Autodesk Inventor part; units mm, degrees
ref_plane "YZ Plane" through (0, 0, 0) normal (1, 0, 0) x (0, 1, 0)
ref_plane "XZ Plane" through (0, 0, 0) normal (0, 1, 0) x (-1, 0, 0)
ref_plane "XY Plane" through (0, 0, 0) normal (0, 0, 1) x (1, 0, 0)
sketch "Sketch1" plane through (0, 0, 0) normal (0, 1, 0) x (-1, 0, 0)
  circle A0 centre (59.0549, -74.4145) radius 1.6
  circle A1 centre (-59.0549, -74.4145) radius 1.6
  line L0 (57.79, -78.2092) -> (0, -58.9459)
  line L1 (-57.79, -78.2092) -> (0, -58.9459)
  line L2 (-60.3198, -70.6198) -> (0, -50.5132)
  line L3 (60.3198, -70.6198) -> (0, -50.5132)
  arc A2 (57.79, -78.2092) -> (60.3198, -70.6198) centre (59.0549, -74.4145) ccw
  arc A3 (-60.3198, -70.6198) -> (-57.79, -78.2092) centre (-59.0549, -74.4145) ccw
extrude "Extrusion1" add sketch "Sketch1" along normal blind 45
properties part number "Front Support"
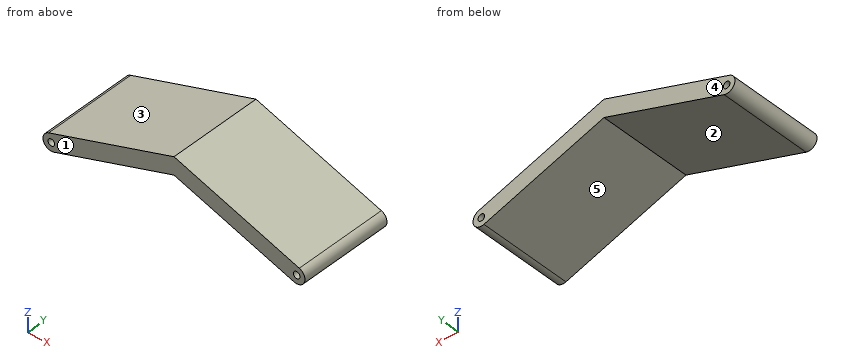
Design review of the part built by this model. Coordinates are the model's own, in mm. Face numbers are marked on the shaded views. A direction names the side the tool comes from. Round coordinates to 2 decimals unless told otherwise and drop trailing zeros. Write each loop counter-clockwise with the first axis right and the second up, starting at its lowest first coordinate (ties: lowest second). Pieces come first, ordered by that corner, then holes. Notation, with made-up numbers: (42.25, -7.75) -> (101.25, -7.75) arc R9 ccw to (101.25, -1.75) -> close; hole circle Ø6 at (35, 75). An arc over 180 degrees is marked (long way). One line per question, with ' | ' between items.
(1) Take a section at A-A, the plane z = -67.75. State the section outline as (x, y) points, and give its area (3 significant figures).
Result sheet:
outline: (-51.71, 0) -> (-26.41, 0) -> (-26.41, 45) -> (-51.71, 45) -> close; (26.41, 0) -> (51.71, 0) -> (51.71, 45) -> (26.41, 45) -> close | area: 2,280 mm2
(2) Wall thickness on line 1 (Z direction, x = 27.5, y = 32.5); line 2 (Z direction, x = -29, y = 35): over which ranges is each line inside the solid? List them lowest first. Write a range as [from, to].
Result sheet:
line 1: [-68.11, -59.68] | line 2: [-68.61, -60.18]
(3) Draft analysis for pull direction X (two halves, no side actions). For the marked faces 1, 2 and 3, state which applies: released by +X, released by -X, zero draft, split by the parting line, or undercut.
Result sheet:
face 1: zero draft | face 2: undercut | face 3: released by -X
(4) Machinability: for the marked faces 4 and 5, which of the approach directions +Z, -Z, +X, -X, +Y, -Y give a long, thin tool a straight path to every point of the face, cutting with its end or side? Answer none if there is none.
Result sheet:
face 4: +Z, -Z, +X, -X, +Y | face 5: -Z, +Y, -Y
(5) Take a section at D-D, the plane z = -56.25. State the section outline as (x, y) points.
Result sheet:
outline: (-17.21, 0) -> (17.21, 0) -> (17.21, 45) -> (-17.21, 45) -> close
(6) Take a section at B-B, the plane y = 10. State the section outline as (x, z) points, and give its area (3 significant figures).
Result sheet:
outline: (-60.32, -70.62) arc R4 ccw to (-57.79, -78.21) -> (0, -58.95) -> (57.79, -78.21) arc R4 ccw to (60.32, -70.62) -> (0, -50.51) -> close; hole circle Ø3.2 at (-59.05, -74.41); hole circle Ø3.2 at (59.05, -74.41) | area: 1,030 mm2
(7) Take a section at C-C, the plane x = -44. State the section outline as (y, z) points, and give its area (3 significant figures).
Result sheet:
outline: (0, -73.61) -> (45, -73.61) -> (45, -65.18) -> (0, -65.18) -> close | area: 379 mm2
(8) Insertion check: P1, Ø3.5, axis at x = 59.05, z = -74.41, coming from the +Y side; P2, Ø1.5, axis at x = 4, y = 29, coming from the +Z side; P3, Ø1.5, axis at x = 37, z = -74, coming from the -Y side; P4, Ø6, axis at y = 39.5, z = -70, coming from the +X side. Each pin has a flat end and moves straight along its axis. Give the tip position at first contact, or say it passes through.
Result sheet:
P1: y = 45 | P2: z = -51.6 | P3: through | P4: x = 62.8
